from build123d import *

# Parameters (mm, degrees)
SKETCH1_R           = 11
BOSS_EXTRUDE1_DEPTH = 7


with BuildPart() as part:
    # Sketch1 → Boss-Extrude1 (new body)
    with BuildSketch(Plane.XY):
        with BuildLine():
            ThreePointArc((16, 25), (0, 41), (-16, 25))
            Line((-16, 25), (-16, -25))
            ThreePointArc((-16, -25), (0, -41), (16, -25))
            Line((16, -25), (16, 25))
        make_face()
        with Locations((0, 25)):
            Circle(SKETCH1_R, mode=Mode.SUBTRACT)
        with Locations((0, -25)):
            Circle(SKETCH1_R, mode=Mode.SUBTRACT)
    extrude(amount=BOSS_EXTRUDE1_DEPTH)


solid = part.part
Design review of the part built by this model. Coordinates are the model's own, in mm. Round coordinates to 2 decimals unless told otherwise and drop trailing zeros. Order: outer loops, then holes, each group sorted by start corner. A loop starts at its lowest first (then second) coordinate and runs counter-clockwise, first axis right, second up.
1) Consider section A-A (x = 0). State the section outline as (y, z) points, plus the area to 3 significant figures.
The answers:
outline: (-41, 0) - (-36, 0) - (-36, 7) - (-41, 7) - close; (-14, 0) - (14, 0) - (14, 7) - (-14, 7) - close; (36, 0) - (41, 0) - (41, 7) - (36, 7) - close
area: 266 mm2
2) Consider section B-B (z = 5.5). State the section outline as (x, y) points, plus the area to 3 significant figures.
The answers:
outline: (-16, -25) arc R16 ccw to (16, -25) - (16, 25) arc R16 ccw to (-16, 25) - close; hole circle Ø22 at (0, -25); hole circle Ø22 at (0, 25)
area: 1,640 mm2
3) Consider section C-C (y = -28). State the section outline as (x, z) points.
The answers:
outline: (-15.72, 0) - (-10.58, 0) - (-10.58, 7) - (-15.72, 7) - close; (10.58, 0) - (15.72, 0) - (15.72, 7) - (10.58, 7) - close
4) For L1, parallel to Y at x = 0, z = 5.5; L2, parallel to Y at x = 1.5, z = 1.5; L3, parallel to X at y = 28.5, z = 5, list the stretches that pass through material, from the lowest coordinate up.
The answers:
L1: y = -41 to -36, -14 to 14, 36 to 41
L2: y = -40.93 to -35.9, -14.1 to 14.1, 35.9 to 40.93
L3: x = -15.61 to -10.43, 10.43 to 15.61
5) Consider section D-D (y = 26.5). State the section outline as (x, z) points, plus the area to 3 significant figures.
The answers:
outline: (-15.93, 0) - (-10.9, 0) - (-10.9, 7) - (-15.93, 7) - close; (10.9, 0) - (15.93, 0) - (15.93, 7) - (10.9, 7) - close
area: 70.5 mm2
6) Clearance check with flat-ended pins moving along their axes: pin 1 Ø17.5 at (x, y) = (0, 25) entering from +Z; pin 2 Ø4 at (x, z) = (11, 3) entering from +Y; pin 3 Ø2 at (x, y) = (-10.5, 5.5) entering from -Z; pin 4 Ø1 at (y, z) = (-32.5, 5) entering from -X. State where each tip first meets the part, or that it passes through.
The answers:
pin 1: passes through
pin 2: stops at y = 38.23
pin 3: stops at z = 0
pin 4: stops at x = -14.39
7) Draft analysis for pull direction Y (two halves, no side actions). For faces 1 (the cylindrical face through (0, 41, 3)), 2 (the cylindrical face through (-2.38, -35.74, 3.45)), 3 (the cylindrical face through (-2.38, 14.26, 3.45)), 4 (the flat face through (-16, 0, 3)), state which applies: released by +Y, released by -Y, zero draft, split by the parting line, or undercut.
The answers:
face 1: released by +Y
face 2: undercut
face 3: undercut
face 4: zero draft
